```python
from build123d import *

# Parameters (mm, degrees)
SKETCH_2_R                      = 25
SKETCH_2_R_2                    = 17.5
EXTRUDE_1_DEPTH                 = 38
SKETCH_3_R                      = 7.5
EXTRUDE_2_DEPTH                 = 15
CUT_EXTRUDE_START               = 70
SKETCH_4_W                      = 76
SKETCH_4_H                      = 4
CUT_EXTRUDE_1_DEPTH             = 64.018795664
EXTRUDE_3_DEPTH                 = 25
EXTRUDE_4_DEPTH                 = 5
SKETCH_5_6_R                    = 19
SKETCH_5_6_R_2                  = 12.5
EXTRUDE_5_DEPTH                 = 32
EXTRUDE_6_REACH                 = 224.284
EXTRUDE_6_END_RADIUS            = 19
SKETCH_7_R                      = 11
SKETCH_7_R_2                    = 7.5
CUT_EXTRUDE_2_REACH             = 224.284
SKETCH_7_2_R                    = 7.5
CUT_EXTRUDE_3_REACH             = 194.608
SKETCH_8_R                      = 17.5
CUT_EXTRUDE_3_DIRECTION_2_DEPTH = 193.608411122


with BuildPart() as part:
    # 草图2 → 凸台-拉伸1 (new, symmetric)
    with BuildSketch(Plane(origin=(0, 0, 0), x_dir=(0, 0, -1), z_dir=(1, 0, 0))):
        with Locations((0, 70)):
            Circle(SKETCH_2_R)
        with Locations((0, 70)):
            Circle(SKETCH_2_R_2, mode=Mode.SUBTRACT)
    extrude(amount=EXTRUDE_1_DEPTH, both=True)

    # 草图3 → 凸台-拉伸2 (add, symmetric)
    with BuildSketch(Plane.XY):
        with BuildLine():
            Line((-15, 110), (-15, 87.5))
            Line((-15, 87.5), (15, 87.5))
            Line((15, 87.5), (15, 110))
            ThreePointArc((15, 110), (0, 125), (-15, 110))
        make_face()
        with Locations((0, 110)):
            Circle(SKETCH_3_R, mode=Mode.SUBTRACT)
    extrude(amount=EXTRUDE_2_DEPTH, both=True)

    # 草图4 → 切除-拉伸1 (cut, through all)
    with BuildSketch(Plane(origin=(0, 0, 0), x_dir=(1, 0, 0), z_dir=(0, 1, 0)).offset(CUT_EXTRUDE_START)):
        Rectangle(SKETCH_4_W, SKETCH_4_H)
    extrude(amount=CUT_EXTRUDE_1_DEPTH, mode=Mode.SUBTRACT)

    # 草图5 → 凸台-拉伸3 (add, symmetric)
    with BuildSketch(Plane.XY):
        with BuildLine():
            Line((-28, 5), (-99.66969722, 5))
            ThreePointArc((-99.66969722, 5), (-99.168168533, 2.522325037), (-99, 0))
            ThreePointArc((-99, 0), (-99.168168533, -2.522325037), (-99.66969722, -5))
            Line((-99.66969722, -5), (-28, -5))
            ThreePointArc((-28, -5), (-17.393398282, -0.606601718), (-13, 10))
            Line((-13, 10), (-13, 70))
            Line((-13, 70), (-23, 70))
            Line((-23, 70), (-23, 10))
            ThreePointArc((-23, 10), (-24.464466094, 6.464466094), (-28, 5))
        make_face()
    extrude(amount=EXTRUDE_3_DEPTH, both=True)

    # 草图5<5> → 凸台-拉伸4 (add, symmetric)
    with BuildSketch(Plane.XY):
        with BuildLine():
            ThreePointArc((-99.66969722, -5), (-106.467437405, -15.099668871), (-118, -19))
            Line((-118, -19), (-7, -19))
            ThreePointArc((-7, -19), (21.284271247, -7.284271247), (33, 21))
            Line((33, 21), (33, 70))
            Line((33, 70), (-13, 70))
            Line((-13, 70), (-13, 10))
            ThreePointArc((-13, 10), (-17.393398282, -0.606601718), (-28, -5))
            Line((-28, -5), (-99.66969722, -5))
        make_face()
    extrude(amount=EXTRUDE_4_DEPTH, both=True)

    # 草图5<6> → 凸台-拉伸5 (add, symmetric)
    with BuildSketch(Plane.XY):
        with Locations((-118, 0)):
            Circle(SKETCH_5_6_R)
        with Locations((-118, 0)):
            Circle(SKETCH_5_6_R_2, mode=Mode.SUBTRACT)
    extrude(amount=EXTRUDE_5_DEPTH, both=True)

    # 凸台-拉伸6: up to this cylinder (the profile starts outside it)
    extrude_6_end = Plane(origin=(-118, 0, -10.688873), z_dir=(0, 0, -1)) * Cylinder(EXTRUDE_6_END_RADIUS, 487.568, mode=Mode.PRIVATE)
    # 草图7 → 凸台-拉伸6 (add, up to the surface)
    with BuildSketch(Plane.ZY.offset(143), mode=Mode.PRIVATE) as extrude_6_sk1:
        Circle(SKETCH_7_R)
        Circle(SKETCH_7_R_2, mode=Mode.SUBTRACT)
    extrude_6_tool1 = extrude(extrude_6_sk1.sketch, amount=-EXTRUDE_6_REACH, mode=Mode.PRIVATE) - extrude_6_end
    add(extrude_6_tool1.solids().sort_by_distance((-143, 0, -10.688873))[0])

    # 草图7<2> → 切除-拉伸2 (cut, up to next)
    with BuildSketch(Plane.ZY.offset(143), mode=Mode.PRIVATE) as cut_extrude_2_sk1:
        Circle(SKETCH_7_2_R)
    cut_extrude_2_tool1 = extrude(cut_extrude_2_sk1.sketch, amount=-CUT_EXTRUDE_2_REACH, mode=Mode.PRIVATE) & part.part
    add(cut_extrude_2_tool1.solids().sort_by_distance((-143, 0, 0))[0], mode=Mode.SUBTRACT)

    # 草图8 → 切除-拉伸3 (cut, up to next)
    with BuildSketch(Plane(origin=(0, 0, 0), x_dir=(0, 0, -1), z_dir=(1, 0, 0)), mode=Mode.PRIVATE) as cut_extrude_3_sk1:
        with Locations((0, 70)):
            Circle(SKETCH_8_R)
    cut_extrude_3_tool1 = extrude(cut_extrude_3_sk1.sketch, amount=-CUT_EXTRUDE_3_REACH, mode=Mode.PRIVATE) & part.part
    add(cut_extrude_3_tool1.solids().sort_by_distance((0, 70, 0))[0], mode=Mode.SUBTRACT)

    # 草图8 → 切除-拉伸3 direction 2 (cut)
    with BuildSketch(Plane(origin=(0, 0, 0), x_dir=(0, 0, -1), z_dir=(1, 0, 0))):
        with Locations((0, 70)):
            Circle(SKETCH_8_R)
    extrude(amount=CUT_EXTRUDE_3_DIRECTION_2_DEPTH, mode=Mode.SUBTRACT)


solid = part.part
```
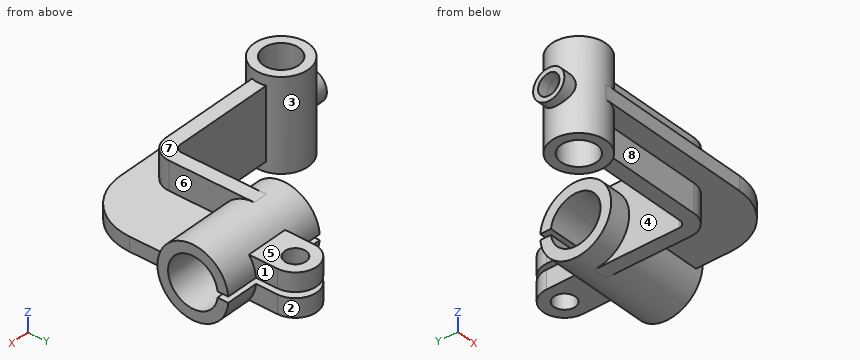
Geometry check sheet. Reference: the model listing, model coordinates, mm. Face numbers are marked on the shaded views. A direction names the side the tool comes from. Coordinates: 2 decimals unless noted, no trailing zeros. Write each loop counter-clockwise with the first axis right and the second up, starting at its lowest first coordinate (ties: lowest second). Pieces come first, ordered by that corner, then holes. Notation, with made-up numbers: (33.5, -35) -> (86.5, -35) arc R19 ccw to (86.5, -14) -> close; hole circle Ø9 at (58.25, 24). An arc over 180 degrees is marked (long way). Use CSV: the item, a comma, the result in double quotes. Start each with the question number.
Item 1: Cross-section at B-B, the plane z = 0. Record the cut outline in (x, y).
Item 2: Set-up check for the marked faces 5, 6, 7 and 8: record each of +Z, -Z, +X, -X, +Y, -Y from which the full face is reachable in a straight line by a thin tool's end or side.
Item 3: Cross-section at D-D, the plane y = 36.5. Record the cut outline in (x, z), plus the area to 3 significant figures.
Item 4: Cross-section at A-A, the plane x = -116. Record the cut outline in (y, z), plus the area to 3 significant figures.
Item 5: Mould release check, pull along X, two halves, no side actions. Record for the marked faces 1, 2, 3 and 4: released by +X, released by -X, zero draft, split by the parting line, or undercut.
Item 6: Thickness scan on line 1 (Z direction, x = -17, y = 70); line 2 (Y direction, x = -2.5, z = 10); line 3 (Y direction, x = 0, z = 12.25). Record the ranges inside material, lowest first.
Item 7: Cross-section at C-C, the plane y = 0. Record the cut outline in (x, z).
Item 8: Depth check by flat-ended pin: pin 1 Ø2 at (y, z) = (32.5, 12.5) entering from -X; pin 2 Ø15 at (x, y) = (7.5, 105.5) entering from +Z; pin 3 Ø5 at (y, z) = (36.5, -0.5) entering from +X; pin 4 Ø16 at (y, z) = (50, 15.5) entering from +X. Enter the tip coordinate at first touch or a pass-through.
Answers:
1,outline,"(-143, -11) -> (-133.49, -11) arc R19 ccw to (-118, -19) -> (-7, -19) arc R40 ccw to (33, 21) -> (33, 45) -> (38, 45) -> (38, 52.5) -> (-38, 52.5) -> (-38, 45) -> (-23, 45) -> (-23, 10) arc R5 cw to (-28, 5) -> (-99.67, 5) arc R19 ccw to (-133.49, 11) -> (-143, 11) -> (-143, 7.5) -> (-128, 7.5) arc R12.5 cw (long way) to (-128, -7.5) -> (-143, -7.5) -> close"
2,face 5,"+Z, +X, -X, +Y"
2,face 6,"+Z, +X, -Y"
2,face 7,"+Z, +X, +Y, -Y"
2,face 8,"-Z, +X, -Y"
3,outline,"(-23, -25) -> (-13, -25) -> (-13, -5) -> (33, -5) -> (33, 5) -> (-13, 5) -> (-13, 25) -> (-23, 25) -> close"
3,area,"960 mm^2"
4,outline,"(-19, -5) -> (-18.89, -5) -> (-18.89, -32) -> (-12.34, -32) -> (-12.34, 32) -> (-18.89, 32) -> (-18.89, 5) -> (-19, 5) -> close; (12.34, -32) -> (18.89, -32) -> (18.89, 32) -> (12.34, 32) -> close"
4,area,"840 mm^2"
5,face 1,"released by +X"
5,face 2,"split by the parting line"
5,face 3,"undercut"
5,face 4,"undercut"
6,line 1,"-25 to -17.5, 17.5 to 25"
6,line 2,"47.09 to 55.64, 84.36 to 102.93, 117.07 to 124.79"
6,line 3,"48.21 to 57.5, 82.5 to 102.5, 117.5 to 125"
7,outline,"(-143, -11) -> (-137, -11) -> (-137, -32) -> (-130.5, -32) -> (-130.5, -7.5) -> (-143, -7.5) -> close; (-143, 7.5) -> (-130.5, 7.5) -> (-130.5, 32) -> (-137, 32) -> (-137, 11) -> (-143, 11) -> close; (-105.5, -32) -> (-99, -32) -> (-99, -25) -> (-16.82, -25) -> (-16.82, -5) -> (27.04, -5) -> (27.04, 5) -> (-16.82, 5) -> (-16.82, 25) -> (-99, 25) -> (-99, 32) -> (-105.5, 32) -> close"
8,pin 1,"x = -23"
8,pin 2,"z = 15"
8,pin 3,"x = 33"
8,pin 4,"x = 38"
